Verification items for this drawing (mm, ordinates from the low corner). Give positions to 0.01 mm unless a question says otherwise; leave off trailing zeros. Loops run counter-clockwise (first coordinate to the right, second up) from the corner with the lowest first, then second, coordinate; pieces in that order, holes last. Notation, with made-up numbers: (28.25, -5) -> (49.25, -5) arc R11 ccw to (49.25, 4) -> close; hole circle Ø1 at (7.25, 16). An arc over 180 degrees is marked (long way). Answer as CSV lines item,"result". Start each with the question number.
(1) Gauge pin test, flat end, axial feed: pin 1 Ø1.5 at (x, z) = (42, 35.5) entering from -Y. Record the tip position at first contact, or that the pin passes through.
(2) Section check B-B on x = 25.4. Enter the section's corners in (y, z) (1 decimal).
(3) Section check C-C on y = 1.45. Enter the section's corners in (x, z), plus the area to 3 significant figures.
(4) Section check A-A on z = 25.4. Enter the section's corners in (x, y) (1 decimal).
(5) Material ranges on line 1 (Z direction, x = 25.4, y = 1.8); line 2 (Z direction, x = 25, y = 0.5), recorded low to high. Write a range as from..to.
(6) Section check D-D on z = 39.37. Enter the section's corners in (x, y) (1 decimal), plus the area to 3 significant figures.
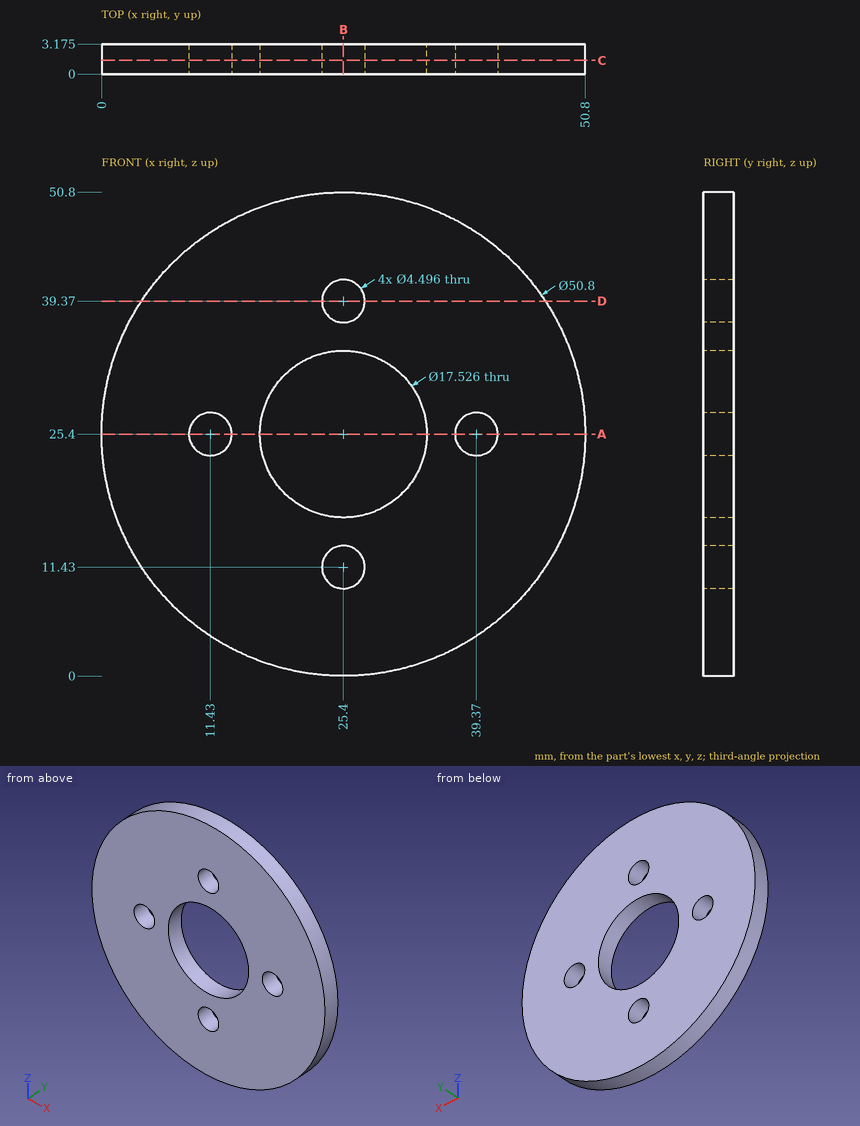
Working result:
1,pin 1,"stops at y = 0"
2,outline,"(0, 0) -> (3.2, 0) -> (3.2, 9.2) -> (0, 9.2) -> close; (0, 13.7) -> (3.2, 13.7) -> (3.2, 16.6) -> (0, 16.6) -> close; (0, 34.2) -> (3.2, 34.2) -> (3.2, 37.1) -> (0, 37.1) -> close; (0, 41.6) -> (3.2, 41.6) -> (3.2, 50.8) -> (0, 50.8) -> close"
3,outline,"circle Ø50.8 at (25.4, 25.4); hole circle Ø4.5 at (11.43, 25.4); hole circle Ø17.53 at (25.4, 25.4); hole circle Ø4.5 at (25.4, 11.43); hole circle Ø4.5 at (25.4, 39.37); hole circle Ø4.5 at (39.37, 25.4)"
3,area,"1,720 mm^2"
4,outline,"(0, 0) -> (9.2, 0) -> (9.2, 3.2) -> (0, 3.2) -> close; (13.7, 0) -> (16.6, 0) -> (16.6, 3.2) -> (13.7, 3.2) -> close; (34.2, 0) -> (37.1, 0) -> (37.1, 3.2) -> (34.2, 3.2) -> close; (41.6, 0) -> (50.8, 0) -> (50.8, 3.2) -> (41.6, 3.2) -> close"
5,line 1,"z = 0..9.18, 13.68..16.64, 34.16..37.12, 41.62..50.8"
5,line 2,"z = 0..9.22, 13.64..16.65, 34.15..37.16, 41.58..50.8"
6,outline,"(4.2, 0) -> (23.2, 0) -> (23.2, 3.2) -> (4.2, 3.2) -> close; (27.6, 0) -> (46.6, 0) -> (46.6, 3.2) -> (27.6, 3.2) -> close"
6,area,"120 mm^2"
